Design review of the part built by this model. Coordinates are the model's own, in mm. A direction names the side the tool comes from. Coordinates: 2 decimals unless noted, no trailing zeros. Write each loop counter-clockwise with the first axis right and the second up, starting at its lowest first coordinate (ties: lowest second). Pieces come first, ordered by that corner, then holes.
Q1. Machinability: for faces 4 (the flat face through (0, 20, 51)), 5 (the flat face through (0, -30, 51)), which of the approach directions +Z, -Z, +X, -X, +Y, -Y give a long, thin tool a straight path to every point of the face, cutting with its end or side? Answer none if there is none.
Q2. Mouldability with a two-part tool opening along X and no side actions: class faces 1 (the flat face through (20, 0, 51)), 2 (the flat face through (-30, 0, 51)), 3 (the flat face through (0, 30, 51)) as pulls with the +X half, pulls with the -X half, needs draft (parallel to the pull), parting line crosses it, or undercut.
Q3. Take a section at B-B (x = -11.5). Give the boundary of the cut face in (y, z).
Q4. For probe 1 along X at (y, z) = (8.5, 44), list the stretches that pass through material, from the lowest coordinate up.
Q5. Insertion check: pin 1 (4 mm diameter, centred on x = -4.5, y = 23.5, fed in from -Z). The pin has a flat end and moves straight along its axis. Give the tip position at first contact, or say it passes through.
Q6. Take a section at A-A (z = 49.5). Give the boundary of the cut face in (x, y).
```python
from build123d import *

# Parameters (mm, degrees)
SKETCH1_W           = 100
SKETCH1_H           = 60
BOSS_EXTRUDE1_DEPTH = 30
SKETCH2_W           = 100
SKETCH2_H           = 40
CUT_EXTRUDE1_DEPTH  = 20


with BuildPart() as part:
    # Sketch1 → Boss-Extrude1 (new, symmetric)
    with BuildSketch(Plane(origin=(0, 0, 0), x_dir=(0, 0, -1), z_dir=(1, 0, 0))):
        with Locations((-50, 0)):
            Rectangle(SKETCH1_W, SKETCH1_H)
    extrude(amount=BOSS_EXTRUDE1_DEPTH, both=True)

    # Sketch2 → Cut-Extrude1 (cut, symmetric)
    with BuildSketch(Plane(origin=(0, 0, 0), x_dir=(0, 0, -1), z_dir=(1, 0, 0))):
        with Locations((-50, 0)):
            Rectangle(SKETCH2_W, SKETCH2_H)
    extrude(amount=CUT_EXTRUDE1_DEPTH, both=True, mode=Mode.SUBTRACT)


solid = part.part
```
Response:
1. face 4: +Z, -Z
1. face 5: +Z, -Z, +X, -X, -Y
2. face 1: undercut
2. face 2: pulls with the -X half
2. face 3: needs draft
3. outline: (-30, 0) - (-20, 0) - (-20, 100) - (-30, 100) - close; (20, 0) - (30, 0) - (30, 100) - (20, 100) - close
4. probe 1: x = -30 to -20, 20 to 30
5. pin 1: stops at z = 0
6. outline: (-30, -30) - (30, -30) - (30, 30) - (-30, 30) - close; hole (-20, -20) - (20, -20) - (20, 20) - (-20, 20) - close
